The model under review builds one solid part; all positions refer to its coordinate system, in mm. A direction names the side the tool comes from. Round coordinates to 2 decimals unless told otherwise and drop trailing zeros. Loops run counter-clockwise (first coordinate to the right, second up) from the corner with the lowest first, then second, coordinate; pieces in that order, holes last. Notation, with made-up numbers: (38, 81.25) - (46, 81.25) arc R22 cw to (46, 104.25) - close; hole circle Ø1 at (74.25, -10.75). An arc over 180 degrees is marked (long way). Answer as CSV lines item,"result".
Autodesk Inventor part; units mm, degrees
ref_plane "YZ Plane" through (0, 0, 0) normal (1, 0, 0) x (0, 1, 0)
ref_plane "XZ Plane" through (0, 0, 0) normal (0, 1, 0) x (-1, 0, 0)
ref_plane "XY Plane" through (0, 0, 0) normal (0, 0, 1) x (1, 0, 0)
sketch "Sketch1" plane through (0, 0, 0) normal (0, 0, 1) x (1, 0, 0)
  circle A0 centre (-15.5, 15.5) radius 1.75
  circle A1 centre (15.5, 15.5) radius 1.75
  circle A2 centre (-15.5, -15.5) radius 1.75
  circle A3 centre (15.5, -15.5) radius 1.75
  circle A4 centre (0, 0) radius 11.05
  line L0 (-15.5, 15.5) -> (15.5, 15.5) construction
  line L1 (15.5, 15.5) -> (15.5, -15.5) construction
  line L2 (15.5, -15.5) -> (-15.5, -15.5) construction
  line L3 (-15.5, -15.5) -> (-15.5, 15.5) construction
  line L4 (-15.5, 15.5) -> (15.5, -15.5) construction
  line L5 (15.5, 15.5) -> (-15.5, -15.5) construction
  line L6 (-25, 25) -> (-25, -25)
  line L7 (-25, -25) -> (25, -25)
  line L8 (25, -25) -> (25, 25)
  line L9 (25, 25) -> (-25, 25)
  dimension "d0" = 22.1
  dimension "d1" = 31
  dimension "d2" = 31
  dimension "d3" = 3.5
  dimension "d4" = 50
  dimension "d5" = 50
extrude "Extrusion1" add sketch "Sketch1" against normal blind 2
sketch "Sketch2" plane through (25, -25, 0) normal (1, 0, 0) x (0, 0, -1)
  line L0 (0, 0) -> (0, 50)
  line L1 (0, 0) -> (2, 0)
  line L2 (2, 50) -> (2, 0)
  line L3 (0, 50) -> (2, 50)
  line L4 (0, 0) -> (0, 50)
  line L5 (0, 59.85) -> (-17.583, 59.85)
  line L6 (-29.1492, 35.2989) -> (0, 0)
  line L7 (0, 38.75) -> (0, 42.25) construction
  line L8 (0, 44.85) -> (-34.6915, 44.85) construction
  line L9 (2, 50) -> (2, 59.85)
  line L10 (2, 59.85) -> (0, 59.85)
  circle A0 centre (-17.583, 44.85) radius 4
  circle A1 centre (-17.583, 44.85) radius 11
  circle A2 centre (-17.583, 44.85) radius 13
  arc A3 (-17.583, 59.85) -> (-29.1492, 35.2989) centre (-17.583, 44.85) ccw
  point P0 (0, 25)
  dimension "d8" = 19.85
  dimension "d9" = 19.583
  dimension "d10" = 8
  dimension "d11" = 22
  dimension "d12" = 2
  dimension "d13" = 2
extrude "Extrusion2" add sketch "Sketch2" against normal blind 7 contours L6 A3 L5 L10 L9 L3 L0 | A2
extrude "Extrusion3" add sketch "Sketch2" along normal blind 1 contours L6 A3 L5 L10 L9 L3 L0 | L0 L3 L2 L1 | A1 | A2
mirror "Mirror1" about plane through (0, 0, 0) normal (1, 0, 0) of "Extrusion2", "Extrusion3"
properties part number "Worm Gear Box" material "PC/ABS Plastic"
1. Take a section at B-B (y = 18). State the section outline as (x, z) points.
Numbers:
outline,"(-26, -2) - (26, -2) - (26, 14.04) - (25, 14.04) - (25, 6.74) - (18, 6.74) - (18, 0) - (-18, 0) - (-18, 6.74) - (-25, 6.74) - (-25, 14.04) - (-26, 14.04) - close; (-26, 21.13) - (-25, 21.13) - (-25, 28.43) - (-18, 28.43) - (-18, 32.47) - (-26, 32.47) - close; (18, 28.43) - (25, 28.43) - (25, 21.13) - (26, 21.13) - (26, 32.47) - (18, 32.47) - close"
2. Take a section at D-D (x = -9.5). State the section outline as (y, z) points.
Numbers:
outline,"(-25, -2) - (-5.64, -2) - (-5.64, 0) - (-25, 0) - close; (5.64, -2) - (25, -2) - (25, 0) - (5.64, 0) - close"
3. Draft analysis for pull direction Z (two halves, no side actions). For faces 1 (the face through (21.549, 30.756, 19.015)), 2 (the face through (22.06, -7.1, 14.78)), 3 (the face through (-2.395, -10.787, -0.986)), 4 (the face through (-25.49, 16.3, 15.74)), state which applies: +Z half, -Z half, draft (parallel to the pull), parting line (faces both ways), or undercut.
Numbers:
face 1,"undercut"
face 2,"+Z half"
face 3,"draft"
face 4,"undercut"
4. Clearance check with flat-ended pins moving along their axes: pin 1 (1.5 mm diameter, centred on x = 18, z = 28.5, fed in from -Y); pin 2 (1.5 mm diameter, centred on x = -5.5, y = 10, fed in from +Z); pin 3 (1 mm diameter, centred on x = 0, z = -0.5, fed in from +Y). State where each tip first meets the part, or that it passes through.
Numbers:
pin 1,"stops at y = 8.6"
pin 2,"stops at z = 0"
pin 3,"stops at y = 25"
5. Take a section at C-C (z = 25). State the section outline as (x, y) points, plus the area to 3 significant figures.
Numbers:
outline,"(-26, 5.27) - (-18, 5.27) - (-18, 11.73) - (-25, 11.73) - (-25, 27.97) - (-18, 27.97) - (-18, 32.89) - (-26, 32.89) - close; (18, 5.27) - (26, 5.27) - (26, 32.89) - (18, 32.89) - (18, 27.97) - (25, 27.97) - (25, 11.73) - (18, 11.73) - close"
area,"214 mm²"
6. Take a section at A-A (x = 15.5). State the section outline as (y, z) points, plus the area to 3 significant figures.
Numbers:
outline,"(-25, -2) - (-17.25, -2) - (-17.25, 0) - (-25, 0) - close; (-13.75, -2) - (13.75, -2) - (13.75, 0) - (-13.75, 0) - close; (17.25, -2) - (25, -2) - (25, 0) - (17.25, 0) - close"
area,"86.0 mm²"
7. Tool access review of faces 5 (the face through (0, 25, -1)), 6 (the face through (-25, 15, 17)), 7 (the face through (15.272, -13.765, -0.986)): name each direction out of +Z, -Z, +X, -X, +Y, -Y from which nothing blocks a thin tool from reaching the whole face with its end or side.
Numbers:
face 5,"+Z, -Z, +Y"
face 6,"none"
face 7,"+Z, -Z"
8. Wall thickness on probe 1 along X at (y, z) = (2.5, 6.5); probe 2 along Y at (x, z) = (-15, -1); probe 3 along X at (y, z) = (29.5, 19): over which ranges is each line inside the solid? List them lowest first.
Numbers:
probe 1,"x = -26 to -18, 18 to 26"
probe 2,"y = -25 to -17.18, -13.82 to 13.82, 17.18 to 25"
probe 3,"x = -26 to -25, 25 to 26"
